Model file for the job. Use its own axes, mm. Give positions to 0.01 mm unless a question says otherwise; leave off trailing zeros. Write each loop counter-clockwise with the first axis right and the second up, starting at its lowest first coordinate (ties: lowest second). Pieces come first, ordered by that corner, then holes. Notation, with made-up numbers: (-17.5, 74) - (19.5, 74) arc R20 ccw to (19.5, 104) - close; hole circle Ø11 at (70.5, -27). An arc over 180 degrees is marked (long way). Use a Markdown table: item, result. Add a question column.
```python
from build123d import *

# Parameters (mm, degrees)
EXTRUDE_4_OUTLINE_R   = 1.1
EXTRUDE_4_OUTLINE_R_2 = 1.75
EXTRUDE_4_DEPTH       = 3
EXTRUDE_START         = 2
EXTRUDE_5_DEPTH       = 2
SKETCH_3_R            = 4
SKETCH_3_R_2          = 1.5
EXTRUDE_6_DEPTH       = 12
EXTRUDE_7_DEPTH       = 3


# Read off the part's stored shape, not the designer's step: 填料-伸長4
with BuildPart() as part:
    # 填料-伸長4 outline → 填料-伸長4 (new body)
    with BuildSketch(Plane(origin=(0, 14.156954032, 0), x_dir=(1, 0, 0), z_dir=(0, 1, 0))):
        with BuildLine():
            Line((-47.225195315, -232.018106976), (-52.72903426, -219.575471046))
            ThreePointArc((-52.72903426, -219.575471046), (-62.201062568, -213.623339578), (-62.862967802, -224.790661134))
            Line((-62.862967802, -224.790661134), (-55.936861757, -236.501360817))
            ThreePointArc((-55.936861757, -236.501360817), (-49.388610218, -238.519947074), (-47.225195315, -232.018106976))
        make_face()
        with Locations((-52.271411996, -232.918210387)):
            Circle(EXTRUDE_4_OUTLINE_R, mode=Mode.SUBTRACT)
        with Locations((-54.193279849, -229.183719263)):
            Circle(EXTRUDE_4_OUTLINE_R, mode=Mode.SUBTRACT)
        with Locations((-59.226743272, -219.402909175)):
            Circle(EXTRUDE_4_OUTLINE_R_2, mode=Mode.SUBTRACT)
        with Locations((-56.115147701, -225.449228139)):
            Circle(EXTRUDE_4_OUTLINE_R, mode=Mode.SUBTRACT)
    extrude(amount=EXTRUDE_4_DEPTH)

    # 草圖2 → 填料-伸長5 (add)
    with BuildSketch(Plane.XZ.offset(-14.156954032).offset(EXTRUDE_START)):
        with BuildLine():
            Line((-52.72903426, 219.575471046), (-47.225195315, 232.018106976))
            ThreePointArc((-47.225195315, 232.018106976), (-49.388610218, 238.519947074), (-55.936861757, 236.501360817))
            Line((-55.936861757, 236.501360817), (-62.862967802, 224.790661134))
            ThreePointArc((-62.862967802, 224.790661134), (-62.201062567, 213.623339578), (-52.72903426, 219.575471046))
        make_face()
        with BuildLine():
            Line((-54.758018868, 219.932533757), (-49.037497118, 232.865028725))
            ThreePointArc((-49.037497118, 232.865028725), (-50.303785386, 236.741617967), (-54.194327422, 235.518869919))
            Line((-54.194327422, 235.518869919), (-61.393110067, 223.347127084))
            ThreePointArc((-61.393110067, 223.347127084), (-61.2858874, 215.401668685), (-54.758018868, 219.932533757))
        make_face(mode=Mode.SUBTRACT)
    extrude(amount=-EXTRUDE_5_DEPTH)

    # 草圖3 → 填料-伸長6 (add)
    with BuildSketch(Plane(origin=(0, 17.156954032, 0), x_dir=(1, 0, 0), z_dir=(0, 1, 0))):
        with Locations(Location((-59.226743272, -219.402909175, 0), (0, 0, 270))):
            Circle(SKETCH_3_R)
        with Locations(Location((-59.226743272, -219.402909175, 0), (0, 0, 270))):
            Circle(SKETCH_3_R_2, mode=Mode.SUBTRACT)
    extrude(amount=EXTRUDE_6_DEPTH)

    # 草圖4 → 填料-伸長7 (add)
    with BuildSketch(Plane(origin=(0, 29.156954032, 0), x_dir=(1, 0, 0), z_dir=(0, 1, 0))):
        with BuildLine():
            Line((-57.061762074, -216.03945018), (18.616065321, -264.75152713))
            Line((18.616065321, -264.75152713), (14.286102925, -271.478445121))
            Line((14.286102925, -271.478445121), (-61.39172447, -222.766368171))
            ThreePointArc((-61.39172447, -222.766368171), (-62.590202267, -217.237927978), (-57.061762074, -216.03945018))
        make_face()
    extrude(amount=EXTRUDE_7_DEPTH)


solid = part.part
```
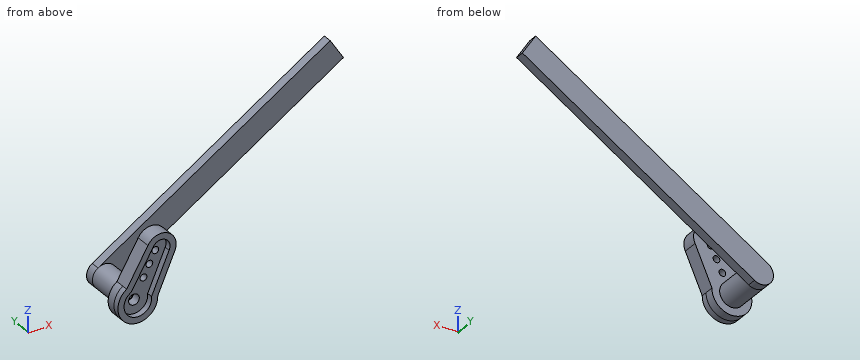
(1) Band-saw the part on A-A (y = 30.5). Write the cut outline in (x, z), then the cut area to 3 significant figures.
(2) Flat gauge pins, fed straight in: pin 1 (2 mm diameter, centred on x = -56.12, z = 225.45, fed in from -Y); pin 2 (3 mm diameter, centred on x = -58.5, z = 218.5, fed in from -Y); pin 3 (2 mm diameter, centred on y = 15.5, z = 236.5, fed in from -X). Where does each tip first touch, or does it go through?
(3) Band-saw the part on B-B (z = 257). Write the cut outline in (x, y), then the cut area to 3 significant figures.
(4) Probe probe 1 along Y at (x, z) = (-50.5, 220.5); probe 2 along X at (y, z) = (17, 225); probe 3 along Y at (x, z) = (-58, 230.5). List the from-to ranges inside material, lowest first. Write a range as [from, to].
(5) Band-saw the part on C-C (y = 26.25). Write the cut outline in (x, z).
Model answer:
| question | item | result |
|---|---|---|
| 1 | outline | (-61.39, 222.77) arc R4 ccw to (-57.06, 216.04) - (18.62, 264.75) - (14.29, 271.48) - close |
| 1 | area | 745 mm^2 |
| 2 | pin 1 | stops at y = 29.16 |
| 2 | pin 2 | stops at y = 14.16 |
| 2 | pin 3 | stops at x = -56.53 |
| 3 | outline | (-8.21, 29.16) - (6.57, 29.16) - (6.57, 32.16) - (-8.21, 32.16) - close |
| 3 | area | 44.3 mm^2 |
| 4 | probe 1 | y = [29.16, 32.16] |
| 4 | probe 2 | x = [-62.74, -57.12], [-55.11, -50.33] |
| 4 | probe 3 | y = [12.16, 17.16] |
| 5 | outline | circle Ø8 at (-59.23, 219.4); hole circle Ø3 at (-59.23, 219.4) |
